from build123d import *

# Parameters (mm, degrees)
F0_R     = 11.6967557634
F0_R_2   = 19.05
F0_R_3   = 6.35
F1_DEPTH = 25.4
F2_DEPTH = 50.8
F3_SIZE  = 5.08


with BuildPart() as f1:
    # F0 (on Top) → F1 (new body)
    with BuildSketch(Plane.XY):
        with BuildLine():
            Line((92.4426392051, -33.1271603522), (92.4426392051, 119.0881550823))
            Line((92.4426392051, 119.0881550823), (11.4402162096, 119.0881550823))
            Line((11.4402162096, 119.0881550823), (11.4402162096, 21.4330990914))
            Line((11.4402162096, 21.4330990914), (-103.7965849838, 21.4330990914))
            ThreePointArc((-103.7965849838, 21.4330990914), (-191.1610406822, -5.8470306304), (-103.7965849838, -33.1271603522))
            Line((-103.7965849838, -33.1271603522), (92.4426392051, -33.1271603522))
        make_face()
        with Locations((-143.2196122709, -5.8470306304)):
            Circle(F0_R, mode=Mode.SUBTRACT)
        with Locations((48.7039178401, 60.5212869929)):
            Circle(F0_R_2, mode=Mode.SUBTRACT)
        with Locations((48.7039178401, 60.5212869929)):
            Circle(F0_R_2)
        with Locations((-143.2196122709, -5.8470306304)):
            Circle(F0_R)
        with Locations((-143.2196122709, -5.8470306304)):
            Circle(F0_R_3, mode=Mode.SUBTRACT)
    extrude(amount=F1_DEPTH)

    # F0 (on Top) → F2 (join)
    with BuildSketch(Plane.XY):
        with Locations((-143.2196122709, -5.8470306304)):
            Circle(F0_R)
        with Locations((-143.2196122709, -5.8470306304)):
            Circle(F0_R_3, mode=Mode.SUBTRACT)
        with Locations((48.7039178401, 60.5212869929)):
            Circle(F0_R_2)
    extrude(amount=F2_DEPTH)

    # F3
    f3_edges = [f1.edges().sort_by_distance(p)[0] for p in [
        (29.653918, 60.521287, 50.8),
        (-154.916368, -5.847031, 25.4),
        (-154.916368, -5.847031, 50.8),
        (29.653918, 60.521287, 25.4),
    ]]
    chamfer(f3_edges, length=F3_SIZE)


solid = f1.part
Here's how the part is built. I have some questions about the finished solid (model axes, mm). A direction names the side the tool comes from. Round coordinates to 2 decimals unless told otherwise and drop trailing zeros. Loops run counter-clockwise (first coordinate to the right, second up) from the corner with the lowest first, then second, coordinate; pieces in that order, holes last. Notation, with made-up numbers: M 59.25,-8 L 87.25,-8 A11 ccw 87.25,-1 Z; hole C -19.75,53.5 d5. An arc over 180 degrees is marked long. Write each question's results on one line, items separated by ' | '. Start each with the question number.
(1) I want a section at B-B (z = 9.5). Please give me the cut outline in (x, y), then the cut area to 3 significant figures.
(2) I want a section at D-D (x = -171). Please give me the cut outline in (y, z).
(3) Will these pins go through, and if not, where does the flat tip stop? P1, Ø4, axis at x = 34, z = 30.5, coming from the +Y side; P2, Ø2, axis at x = 19, z = 22.5, coming from the -Y side; P3, Ø12, axis at x = 60, y = -5, coming from the +Z side; P4, Ø10, axis at x = -56, y = -36.5, coming from the -Z side.
(4) On a 3-axis mill with a long thin cutter (end or side, diameter ignored), from which of +Z, -Z, +X, -X, +Y, -Y can I reach the whole of each face in a straight line? I mean faces 4 (the cylindrical face through (44.574, 41.924, 37.993)), 5 (the flat face through (11.44, 71, 13)), 6 (the flat face through (49, 61, 50.8)), 7 (the flat face through (-20, 15, 0)), 8 (the flat face through (-7, -33.127, 13)). Say none if no direction works.
(5) If I drill on probe 1 along Z at (x, y) = (-22.5, -28.5); probe 2 along X at (y, z) = (47.5, 14.5); probe 3 along Y at (x, z) = (-54.5, 4.5), over which ranges is the centre line in solid material (lowest first)? Write a range as from..to.
(6) I want a section at A-A (z = 43). Please give me the cut outline in (x, y).
(7) I want a section at C-C (x = -62.5). Please give me the cut outline in (y, z).
(8) Thinking about a two-plate mould opening in X: for faces 1 (the flat face through (92.443, 42, 13)), 2 (the cylindrical face through (-132.063, -2.334, 37.993)), 3 (the flat face through (-45, 21.433, 13)), which applies, pulls with the +X half, pulls with the -X half, needs draft (parallel to the pull), parting line crosses it, or undercut?
Solved:
1) outline: M -103.8,-33.13 L 92.44,-33.13 L 92.44,119.09 L 11.44,119.09 L 11.44,21.43 L -103.8,21.43 A47.94 ccw long Z; hole C -143.22,-5.85 d12.7 | area: 25,400 mm²
2) outline: M -44.92,0 L 33.23,0 L 33.23,25.4 L -44.92,25.4 Z
3) P1: stops at y = 76.12 | P2: stops at y = -33.13 | P3: stops at z = 25.4 | P4: stops at z = 0
4) face 4: +Z | face 5: +Z, -Z, +Y | face 6: +Z, +X, -X, +Y, -Y | face 7: -Z, +X, -X, +Y, -Y | face 8: +Z, -Z, +X, -Y
5) probe 1: z = 0..25.4 | probe 2: x = 11.44..92.44 | probe 3: y = -33.13..21.43
6) outline: C -143.22,-5.85 d23.39; C 48.7,60.52 d38.1; hole C -143.22,-5.85 d12.7
7) outline: M -33.13,0 L 21.43,0 L 21.43,25.4 L -33.13,25.4 Z
8) face 1: pulls with the +X half | face 2: parting line crosses it | face 3: undercut
